Here's how the part is built. I have some questions about the finished solid (model axes, mm). A direction names the side the tool comes from. Coordinates: 2 decimals unless noted, no trailing zeros. Write each loop counter-clockwise with the first axis right and the second up, starting at its lowest first coordinate (ties: lowest second). Pieces come first, ordered by that corner, then holes. Notation, with made-up numbers: (70.5, -13.5) -> (94.5, -13.5) arc R30 cw to (94.5, 21.5) -> close; hole circle Ø1 at (60.5, 26). An arc over 180 degrees is marked (long way). Put each result on its own line as item: value. Start each with the question number.
Item 1: I need wall thicknesses on line 1 (X direction, y = 9.25, z = -5.5); line 2 (X direction, y = 4, z = 3.25); line 3 (Y direction, x = 49, z = -0.25). Which ranges of each line are inside material? Lowest first, please. Write a range as [from, to].
Item 2: I want a section at C-C, the plane x = 40. List the corners of the cut face in (y, z) for me (3 decimals).
Item 3: If we mould it in two halves opening along Z, with no side actions, what happens to faces 1 (the face through (5.842, -5, 0)), 2 (the face through (7.97, 0.51, -12.69)), 3 (the face through (33, 0, 10.16))? For each: released by +Z, released by -Z, zero draft, split by the parting line, or undercut.
Item 4: For pin 1 (3 mm diameter, centred on x = 58.5, z = -5, fed in from +Y); pin 2 (6.5 mm diameter, centred on x = 1, z = 7.5, fed in from -Y) (3 decimals); pin 3 (7.5 mm diameter, centred on y = -3.5, z = -6, fed in from -X); pin 4 (10 mm diameter, centred on x = 52.5, z = -3.5, fed in from -Y), each with a flat end and sliding along its axis, tell me the tip position at first contact or that it passes through.
Item 5: I want a section at D-D, the plane z = 7.25. List the corners of the cut face in (x, y) for me (3 decimals), then the cut area to 3 significant figures.
Item 6: I want a section at A-A, the plane y = 0. List the corners of the cut face in (x, z) for me, then the cut area to 3 significant figures.
Item 7: On a 3-axis mill with a long thin cutter (end or side, diameter ignored), from which of +Z, -Z, +X, -X, +Y, -Y can I reach the whole of each face in a straight line? I mean faces 4 (the face through (-1.262, -0.044, -6.545)), 5 (the face through (61, 0, 12.7)), 6 (the face through (10.16, 9, 6)). Say none if no direction works.
Item 8: I want a section at B-B, the plane z = 0. List the corners of the cut face in (x, y) for me (3 decimals), then the cut area to 3 significant figures.
from build123d import *

# Parameters (mm, degrees)
F0_W     = 5.842
F0_H     = 12.7
F0_R     = 1.524
F2_DEPTH = 3.175


with BuildPart() as f1:
    # F0 (on Front) → F1 (revolve)
    with BuildSketch(Plane.XZ):
        Polygon((5.842, 12.7), (5.842, 0), (66.294, 0), (66.294, 12.7), (56.134, 12.7), (56.134, 10.16), (10.16, 10.16), (10.16, 12.7), align=None)
    revolve(axis=Axis((33.147, 0, 0), (-1, 0, 0)))

    # F0 (on Front) → F2 (join, symmetric)
    with BuildSketch(Plane.XZ):
        Polygon((5.842, 12.7), (5.842, 0), (66.294, 0), (66.294, 12.7), (56.134, 12.7), (56.134, 10.16), (10.16, 10.16), (10.16, 12.7), align=None)
        with BuildLine():
            Line((-2.5908, 0), (0, 0))
            Line((0, 0), (0, 12.7))
            Line((0, 12.7), (5.842, 12.7))
            Line((5.842, 12.7), (5.842, 15.24))
            Line((5.842, 15.24), (-0.508, 15.24))
            Line((-0.508, 15.24), (-9.9307574264, 2.405036162))
            ThreePointArc((-9.9307574264, 2.405036162), (-5.3893741786, 3.8619675672), (-2.5908, 0))
        make_face()
        with Locations((2.921, 6.35)):
            Rectangle(F0_W, F0_H)
        with BuildLine():
            Line((5.842, 0), (0, 0))
            Line((0, 0), (-2.5908, 0))
            ThreePointArc((-2.5908, 0), (-4.3787043805, -3.3668211611), (-8.1692865802, -3.7712632364))
            Line((-8.1692865802, -3.7712632364), (5.842, -9.398))
            Line((5.842, -9.398), (5.842, 0))
        make_face()
        with BuildLine():
            ThreePointArc((-8.1692865802, -3.7712632364), (-4.3787043805, -3.3668211611), (-2.5908, 0))
            ThreePointArc((-2.5908, 0), (-5.3893741786, 3.8619675672), (-9.9307574264, 2.405036162))
            ThreePointArc((-9.9307574264, 2.405036162), (-10.5629654276, -1.1146026154), (-8.1692865802, -3.7712632364))
        make_face()
        with Locations((-6.6548, 0)):
            Circle(F0_R, mode=Mode.SUBTRACT)
        with Locations((-6.6548, 0)):
            Circle(F0_R)
    extrude(amount=F2_DEPTH, both=True)


solid = f1.part
Calculated:
1. line 1: x = [5.84, 10.16], [56.13, 66.29]
1. line 2: x = [5.84, 66.29]
1. line 3: y = [-10.16, 10.16]
2. outline: (-3.175, 9.651) arc R10.16 ccw (long way) to (3.175, 9.651) -> (3.175, 10.16) -> (-3.175, 10.16) -> close
3. face 1: zero draft
3. face 2: split by the parting line
3. face 3: released by +Z
4. pin 1: stops at y = 12.21
4. pin 2: stops at y = -3.175
4. pin 3: stops at x = -10.03
4. pin 4: stops at y = -12.7
5. outline: (-6.374, -3.175) -> (5.842, -3.175) -> (5.842, -10.427) -> (10.16, -10.427) -> (10.16, -7.118) -> (56.134, -7.118) -> (56.134, -10.427) -> (66.294, -10.427) -> (66.294, 10.427) -> (56.134, 10.427) -> (56.134, 7.118) -> (10.16, 7.118) -> (10.16, 10.427) -> (5.842, 10.427) -> (5.842, 3.175) -> (-6.374, 3.175) -> close
5. area: 1,030 mm2
6. outline: (-9.93, 2.41) arc R4.06 ccw to (-8.17, -3.77) -> (5.84, -9.4) -> (5.84, -12.7) -> (10.16, -12.7) -> (10.16, -10.16) -> (56.13, -10.16) -> (56.13, -12.7) -> (66.29, -12.7) -> (66.29, 12.7) -> (56.13, 12.7) -> (56.13, 10.16) -> (10.16, 10.16) -> (10.16, 12.7) -> (5.84, 12.7) -> (5.84, 15.24) -> (-0.51, 15.24) -> close
6. area: 1,580 mm2
7. face 4: -Z, -X, +Y, -Y
7. face 5: +Z, +X, +Y, -Y
7. face 6: none
8. outline: (-10.719, -3.175) -> (5.842, -3.175) -> (5.842, -12.7) -> (10.16, -12.7) -> (10.16, -10.16) -> (56.134, -10.16) -> (56.134, -12.7) -> (66.294, -12.7) -> (66.294, 12.7) -> (56.134, 12.7) -> (56.134, 10.16) -> (10.16, 10.16) -> (10.16, 12.7) -> (5.842, 12.7) -> (5.842, 3.175) -> (-10.719, 3.175) -> close
8. area: 1,410 mm2
